```python
from build123d import *

# Parameters (mm, degrees)
ESQUISSE1_R                  = 50
ESQUISSE1_R_2                = 11.5
BOSS_EXTRU_1_DEPTH           = 3
ENL_V_MAT_EXTRU_2_DEPTH      = 4
ESQUISSE4_R                  = 1.45
ENL_V_MAT_EXTRU_3_DEPTH      = 71.774289117
R_P_TITION_CIRCULAIRE1_COUNT = 3


with BuildPart() as part:
    # Esquisse1 → Boss.-Extru.1 (new body)
    with BuildSketch(Plane.XY):
        Circle(ESQUISSE1_R)
        Circle(ESQUISSE1_R_2, mode=Mode.SUBTRACT)
    extrude(amount=BOSS_EXTRU_1_DEPTH)

    # Esquisse3 → Enl_v. mat.-Extru.2 (cut)
    with BuildSketch(Plane(origin=(0, 0, 0), x_dir=(-1, 0, 0), z_dir=(0, 0, -1))):
        with BuildLine():
            Line((-50.492676186, 5.5), (-33.753889757, 5.5))
            ThreePointArc((-33.753889757, 5.5), (-28.253889757, 0), (-33.753889757, -5.5))
            Line((-33.753889757, -5.5), (-50.492676186, -5.5))
            ThreePointArc((-50.492676186, -5.5), (-55.992676186, 0), (-50.492676186, 5.5))
        make_face()
        with BuildLine():
            Line((-34.573554166, 19), (-25.753889757, 19))
            ThreePointArc((-25.753889757, 19), (-24.253889757, 17.5), (-25.753889757, 16))
            Line((-25.753889757, 16), (-34.573554166, 16))
            ThreePointArc((-34.573554166, 16), (-36.073554166, 17.5), (-34.573554166, 19))
        make_face()
        with BuildLine():
            Line((-34.573554166, -19), (-25.753889757, -19))
            ThreePointArc((-25.753889757, -19), (-24.253889757, -17.5), (-25.753889757, -16))
            Line((-25.753889757, -16), (-34.573554166, -16))
            ThreePointArc((-34.573554166, -16), (-36.073554166, -17.5), (-34.573554166, -19))
        make_face()
    extrude(amount=-ENL_V_MAT_EXTRU_2_DEPTH, mode=Mode.SUBTRACT)

    # Esquisse4 → Enl_v. mat.-Extru.3 (cut, through all)
    with BuildSketch(Plane.XY):
        with Locations((-45, 0)):
            Circle(ESQUISSE4_R)
    enl_v_mat_extru_3 = extrude(amount=ENL_V_MAT_EXTRU_3_DEPTH, mode=Mode.SUBTRACT)

    # R_p_tition circulaire1: Enl_v. mat.-Extru.3 ×3 about axis
    r_p_tition_circulaire1_axis = Axis((0, 0, 0), (0, 0, 1))
    for i in range(1, R_P_TITION_CIRCULAIRE1_COUNT):
        add(enl_v_mat_extru_3.rotate(r_p_tition_circulaire1_axis, i * 360 / R_P_TITION_CIRCULAIRE1_COUNT), mode=Mode.SUBTRACT)


solid = part.part
```
Geometry: final body of the model. Coordinates: model frame, mm. A direction names the side the tool comes from. Give positions to 0.01 mm unless a question says otherwise; leave off trailing zeros. Loops run counter-clockwise (first coordinate to the right, second up) from the corner with the lowest first, then second, coordinate; pieces in that order, holes last. Notation, with made-up numbers: (-30, -30) -> (5, -30) arc R16 cw to (5, -11) -> close; hole circle Ø3 at (-8.75, 22.25). An arc over 180 degrees is marked (long way). Use CSV: the item, a comma, the result in double quotes.
(1) First-contact query: P1, Ø1.5, axis at x = 30, z = 2, coming from the +Y side; P2, Ø4, axis at x = -26.5, y = -25, coming from the -Z side; P3, Ø1.5, axis at x = 45.5, z = 1, coming from the +Y side; P4, Ø0.9, axis at x = 32, z = 2, coming from the +Y side. Flat tips, straight axial feed; report the tip coordinate or a pass-through.
From the geometry:
P1,"y = 40.55"
P2,"z = 0"
P3,"y = 22.3"
P4,"y = 38.79"
(2) Ray query, line 1 along Y through (x, z) = (0, 2.15); line 2 along X through (y, z) = (-0.5, 2.6); line 3 along Y through (x, z) = (22.5, 1.95). Return the intervals inside material, ascending. Write a range as [from, to].
From the geometry:
line 1,"[-50, -11.5], [11.5, 50]"
line 2,"[-50, -46.36], [-43.64, -11.49], [11.49, 28.28]"
line 3,"[-44.65, -40.42], [-37.52, 37.52], [40.42, 44.65]"
(3) Cut plane C-C (y = -17.5). Output: boundary loops of the cut face in (x, z), plus the area to 3 significant figures.
From the geometry:
outline,"(-46.84, 0) -> (24.25, 0) -> (24.25, 3) -> (-46.84, 3) -> close; (36.07, 0) -> (46.84, 0) -> (46.84, 3) -> (36.07, 3) -> close"
area,"246 mm^2"
(4) Pull-direction query (Y, two-part tool) for faces 1 (the face through (-49.955, 2.121, 1.479)), 2 (the face through (30, 19, 1)), 3 (the face through (-1, 12, 3)), 4 (the face through (42, 5.5, 1)); classes: released by +Y, released by -Y, zero draft, split by the parting line, or undercut.
From the geometry:
face 1,"split by the parting line"
face 2,"undercut"
face 3,"zero draft"
face 4,"undercut"
(5) Access query for faces 5 (the face through (-1, 12, 0)), 6 (the face through (42, -5.5, 1)), 7 (the face through (36.073, 17.467, 1.479)). Directions: +Z, -Z, +X, -X, +Y, -Y. A direction counts if a zero-diameter tool reaches every point of the face in a straight line with its end or side. Return the directions, or none.
From the geometry:
face 5,"-Z, +X, -X, +Y, -Y"
face 6,"+Z, -Z, +X"
face 7,"+Z, -Z"
(6) Cut plane B-B (x = 0). Output: boundary loops of the cut face in (y, z), plus the area to 3 significant figures.
From the geometry:
outline,"(-50, 0) -> (-11.5, 0) -> (-11.5, 3) -> (-50, 3) -> close; (11.5, 0) -> (50, 0) -> (50, 3) -> (11.5, 3) -> close"
area,"231 mm^2"
(7) Cut plane A-A (y = 0). Output: boundary loops of the cut face in (x, z).
From the geometry:
outline,"(-50, 0) -> (-46.45, 0) -> (-46.45, 3) -> (-50, 3) -> close; (-43.55, 0) -> (-11.5, 0) -> (-11.5, 3) -> (-43.55, 3) -> close; (11.5, 0) -> (28.25, 0) -> (28.25, 3) -> (11.5, 3) -> close"
(8) Cut plane D-D (z = 2.5). Output: boundary loops of the cut face in (x, y) (3 decimals).
From the geometry:
outline,"(33.754, -5.5) arc R5.5 cw to (33.754, 5.5) -> (49.697, 5.5) arc R50 ccw (long way) to (49.697, -5.5) -> close; hole circle Ø2.9 at (-45, 0); hole circle Ø23 at (0, 0); hole circle Ø2.9 at (22.5, -38.971); hole circle Ø2.9 at (22.5, 38.971); hole (25.754, -19) -> (34.574, -19) arc R1.5 ccw to (34.574, -16) -> (25.754, -16) arc R1.5 ccw to start; hole (25.754, 16) -> (34.574, 16) arc R1.5 ccw to (34.574, 19) -> (25.754, 19) arc R1.5 ccw to start"
